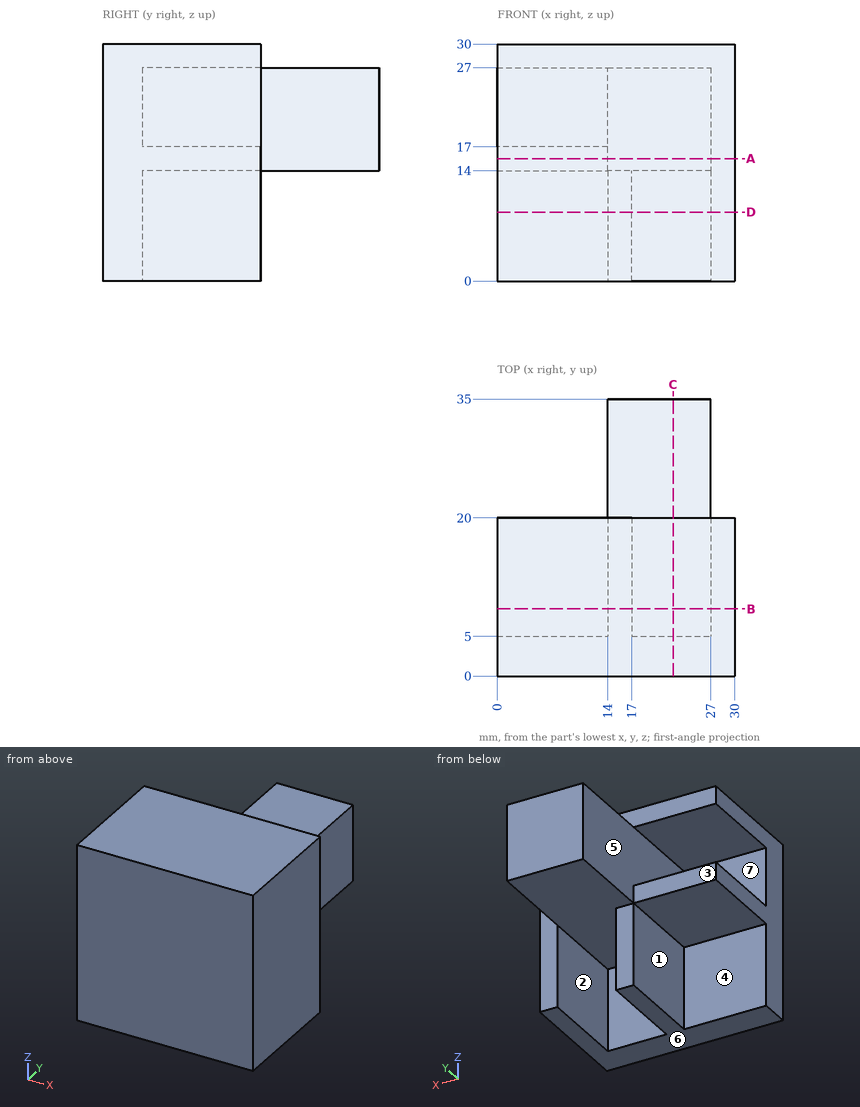
Geometry: see drawing. Coordinates: mm, zero at the bounding-box minimum. A direction names the side the tool comes from. Round coordinates to 2 decimals unless told otherwise and drop trailing zeros. Loops run counter-clockwise (first coordinate to the right, second up) from the corner with the lowest first, then second, coordinate; pieces in that order, holes last. Notation, with made-up numbers: (45, 34) - (54, 34) arc R32 cw to (54, 62) - close; hole circle Ø8 at (16.5, 79.25). An arc over 180 degrees is marked (long way). Use CSV: the item, a comma, the result in double quotes.
Q1. Section query A-A, the plane z = 15.5. Output: boundary loops of the cut face in (x, y), then the cut area to 3 significant figures.
Reported:
outline,"(0, 0) - (30, 0) - (30, 20) - (27, 20) - (27, 35) - (14, 35) - (14, 20) - (0, 20) - close"
area,"795 mm^2"
Q2. Section query D-D, the plane z = 8.75. Output: boundary loops of the cut face in (x, y).
Reported:
outline,"(0, 0) - (30, 0) - (30, 20) - (27, 20) - (27, 5) - (17, 5) - (17, 20) - (14, 20) - (14, 5) - (0, 5) - close"
Q3. Ray query, line 1 along Z through (x, y) = (10, 18); line 2 along Y through (x, z) = (3.5, 11.75). Return the intervals inside material, ascending.
Reported:
line 1,"14 to 17, 27 to 30"
line 2,"0 to 5"
Q4. Mould query, pull axis Z, two halves, no side actions, for the marked faces 4, 5, 6 and 7. Classes: pulls with the +Z half, pulls with the -Z half, needs draft (parallel to the pull), parting line crosses it, or undercut.
Reported:
face 4,"needs draft"
face 5,"undercut"
face 6,"pulls with the -Z half"
face 7,"undercut"
Q5. Pin query (flat end, axial travel): pin 1 Ø2 at (y, z) = (14.5, 20) entering from -X; pin 2 Ø1.5 at (x, z) = (15.5, 4.5) entering from +Y; pin 3 Ø10 at (x, y) = (22.5, 26) entering from +Z; pin 4 Ø4 at (x, z) = (22, 3) entering from -Y. Return the tip coordinate at first contact, or that it passes through.
Reported:
pin 1,"x = 14"
pin 2,"y = 20"
pin 3,"z = 27"
pin 4,"y = 0"
Q6. Section query B-B, the plane y = 8.5. Output: boundary loops of the cut face in (x, z), then the cut area to 3 significant figures.
Reported:
outline,"(0, 14) - (14, 14) - (14, 0) - (17, 0) - (17, 14) - (27, 14) - (27, 0) - (30, 0) - (30, 30) - (0, 30) - (0, 27) - (14, 27) - (14, 17) - (0, 17) - close"
area,"424 mm^2"
Q7. Section query C-C, the plane x = 22.25. Output: boundary loops of the cut face in (y, z), then the cut area to 3 significant figures.
Reported:
outline,"(0, 0) - (5, 0) - (5, 14) - (35, 14) - (35, 27) - (20, 27) - (20, 30) - (0, 30) - close"
area,"585 mm^2"
Q8. Reachability of the marked faces 1, 2 and 3 from +Z, -Z, +X, -X, +Y, -Y: full face, straight path, thin tool, end or side. Return the list, or none.
Reported:
face 1,"-Z, -X, +Y"
face 2,"-Z, +Y"
face 3,"+Z, -Z, -X, +Y"
